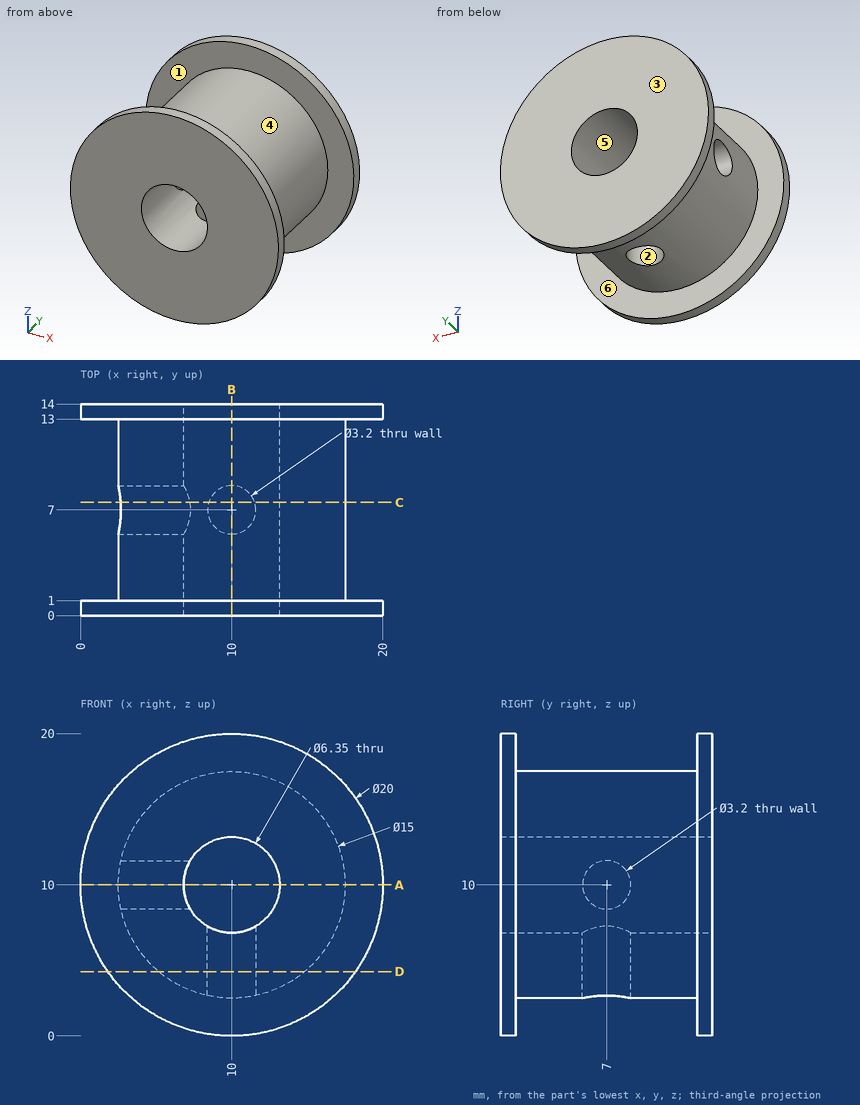
Answer from the drawing. Dimensions are ordinates in mm from the lowest x, y and z of the part. A direction names the side the tool comes from. Give positions to 0.01 mm unless a question says otherwise; leave off trailing zeros. Order: outer loops, then holes, each group sorted by start corner. A loop starts at its lowest first (then second) coordinate and runs counter-clockwise, first axis right, second up. Notation, with made-up numbers: (61.5, 28) - (104.5, 28) arc R24 cw to (104.5, 38) - close; hole circle Ø8 at (19, 53). An arc over 180 degrees is marked (long way). Use one line per item in the form item = value.
1) Consider probe 1 along X at (y, z) = (5.25, 10) (3 decimals); probe 2 along Y at (x, z) = (5.4, 10); probe 3 along Y at (x, z) = (9, 1.5). Determine where each line is inside the solid, lowest interval first. Write a range as [from, to].
Verdict:
probe_1 = [2.5, 6.825], [13.175, 17.5]
probe_2 = [0, 5.4], [8.6, 14]
probe_3 = [0, 1], [13, 14]
2) Find section A-A on z = 10. Determine the outline of the cut face in (x, y) (3 decimals), and give its area (3 significant figures).
Verdict:
outline = (0, 0) - (6.825, 0) - (6.825, 5.4) - (2.5, 5.4) - (2.5, 1) - (0, 1) - close; (0, 13) - (2.5, 13) - (2.5, 8.6) - (6.825, 8.6) - (6.825, 14) - (0, 14) - close; (13.175, 0) - (20, 0) - (20, 1) - (17.5, 1) - (17.5, 13) - (20, 13) - (20, 14) - (13.175, 14) - close
area = 117 mm^2
3) Find section C-C on y = 7.5. Determine the outline of the cut face in (x, z) (3 decimals), and give its area (3 significant figures).
Verdict:
outline = (2.656, 8.48) arc R7.5 ccw to (8.48, 2.656) - (8.48, 7.212) arc R3.175 cw to (7.212, 8.48) - close; (2.656, 11.52) - (7.212, 11.52) arc R3.175 cw (long way) to (11.52, 7.212) - (11.52, 2.656) arc R7.5 ccw (long way) to start
area = 118 mm^2
4) Each of these flat-tipped pins is pushed along its axis until it touches: pin 1 (1.9 mm diameter, centred on y = 7, z = 10, fed in from -X); pin 2 (4 mm diameter, centred on x = 10, y = 7, fed in from -Z); pin 3 (8 mm diameter, centred on y = 6.5, z = 15.5, fed in from -X). Where does it stop, or does it pass through?
Verdict:
pin_1 = 13.03
pin_2 = 2.5
pin_3 = 2.65
5) The mould has two halves that part along X. Classify the marked faces 4, 5 and 6: released by +X, released by -X, zero draft, split by the parting line, or undercut.
Verdict:
face_4 = split by the parting line
face_5 = undercut
face_6 = zero draft
6) Find section D-D on z = 4.25. Determine the outline of the cut face in (x, y).
Verdict:
outline = (1.82, 0) - (18.18, 0) - (18.18, 1) - (14.82, 1) - (14.82, 13) - (18.18, 13) - (18.18, 14) - (1.82, 14) - (1.82, 13) - (5.18, 13) - (5.18, 1) - (1.82, 1) - close; hole circle Ø3.2 at (10, 7)
7) Find section B-B on x = 10. Determine the outline of the cut face in (y, z) (3 decimals), and give its area (3 significant figures).
Verdict:
outline = (0, 0) - (1, 0) - (1, 2.5) - (5.4, 2.5) - (5.4, 6.825) - (0, 6.825) - close; (0, 13.175) - (14, 13.175) - (14, 20) - (13, 20) - (13, 17.5) - (1, 17.5) - (1, 20) - (0, 20) - close; (8.6, 2.5) - (13, 2.5) - (13, 0) - (14, 0) - (14, 6.825) - (8.6, 6.825) - close
area = 117 mm^2
8) For the marked faces 1, 2 and 3, determine the directions among +Z, -Z, +X, -X, +Y, -Y from which every point of the face is accessible in a straight line to the end or side of a thin tool.
Verdict:
face_1 = none
face_2 = -Z
face_3 = +Z, -Z, +X, -X, +Y
